Autodesk Inventor part; units mm, degrees
ref_plane "YZ Plane" through (0, 0, 0) normal (1, 0, 0) x (0, 1, 0)
ref_plane "XZ Plane" through (0, 0, 0) normal (0, 1, 0) x (-1, 0, 0)
ref_plane "XY Plane" through (0, 0, 0) normal (0, 0, 1) x (1, 0, 0)
sketch "Sketch1" plane through (0, 0, 0) normal (0, 1, 0) x (-1, 0, 0)
  line L0 (0, 0) -> (0, 27.94)
  line L1 (71.12, 27.94) -> (71.12, 0)
  arc A0 (49.5914, 27.94) -> (21.5286, 27.94) centre (35.56, 13.97) ccw
  line L2 (0, 27.94) -> (21.5286, 27.94)
  line L3 (49.5914, 27.94) -> (71.12, 27.94)
  circle A1 centre (35.56, 13.97) radius 16.5 construction
  circle A2 centre (35.56, 30.47) radius 1.5
  line L4 (35.56, 13.97) -> (49.8494, 5.72) construction
  line L5 (35.56, 13.97) -> (21.2706, 5.72) construction
  circle A3 centre (21.2706, 5.72) radius 1.5
  circle A4 centre (49.8494, 5.72) radius 1.5
  line L6 (71.12, 13.97) -> (0, 13.97) construction
  line L7 (51.7567, 0) -> (44.8805, 3.97)
  line L8 (19.3633, 0) -> (26.2395, 3.97)
  line L9 (44.8805, 3.97) -> (26.2395, 3.97)
  line L10 (59.055, 13.97) -> (64.775, 13.97) construction
  line L11 (59.055, 11.305) -> (64.775, 11.305)
  line L12 (64.775, 16.635) -> (59.055, 16.635)
  arc A5 (59.055, 16.635) -> (59.055, 11.305) centre (59.055, 13.97) ccw
  arc A6 (64.775, 11.305) -> (64.775, 16.635) centre (64.775, 13.97) ccw
  line L13 (6.33, 13.97) -> (12.08, 13.97) construction
  line L14 (6.33, 11.305) -> (12.08, 11.305)
  line L15 (12.08, 16.635) -> (6.33, 16.635)
  arc A7 (6.33, 16.635) -> (6.33, 11.305) centre (6.33, 13.97) ccw
  arc A8 (12.08, 11.305) -> (12.08, 16.635) centre (12.08, 13.97) ccw
  line L16 (71.12, 0) -> (51.7567, 0)
  line L17 (19.3633, 0) -> (0, 0)
  point P0 (61.915, 13.97)
  point P1 (9.205, 13.97)
  dimension "d0" = 27.94
  dimension "d1" = 71.12
  dimension "d5" = 35.56
  dimension "d7" = 19.8
  dimension "d8" = 33
  dimension "d9" = 3
  dimension "d10" = 3
  dimension "d11" = 3
  dimension "d13" = 30
  dimension "d14" = 4
  dimension "d15" = 4
  dimension "d16" = 10
  dimension "d17" = 2.86
  dimension "d18" = 5.33
  dimension "d19" = 2.875
  dimension "d20" = 5.33
  dimension "d21" = 26.355
  dimension "d22" = 26.355
  dimension "d23" = 13.97
extrude "Extrusion1" add sketch "Sketch1" along normal blind 4.763
fillet "Fillet1" radius 6.35 10 edges at (0, 2.3815, 0) (0, 2.3815, 27.94) (-71.12, 2.3815, 0) (-71.12, 2.3815, 27.94) (-21.5286, 2.3815, 27.94) (-49.5914, 2.3815, 27.94) (-26.2395, 2.3815, 3.97) (-19.3633, 2.3815, 0) (-44.8805, 2.3815, 3.97) (-51.7567, 2.3815, 0)
sketch "Sketch2" plane through (0, 4.763, 0) normal (0, 1, 0) x (1, 0, 0)
  arc A0 (-48.0228, -29.3557) -> (-23.0972, -29.3557) centre (-35.56, -13.97) ccw
  circle A1 centre (-35.56, -13.97) radius 3.4
  point P0 (0, 0)
  dimension "d27" = 6.8
extrude "Extrusion2" cut sketch "Sketch2" against normal blind 3
sketch "Sketch3" plane through (-35.56, 1.763, 13.97) normal (0, 1, 0) x (1, 0, 0)
  circle A0 centre (0, 0) radius 3.4
  circle A1 centre (0, 0) radius 1.75
  point P0 (35.56, 13.97)
  dimension "d30" = 3.5
extrude "Extrusion3" cut sketch "Sketch3" against normal blind 6.75 contours A1
properties part number "MountPlate"
The listing builds one solid part. Answer for the finished solid, in the listing's coordinates (mm). A direction names the side the tool comes from. Round coordinates to 2 decimals unless told otherwise and drop trailing zeros. Order: outer loops, then holes, each group sorted by start corner. A loop starts at its lowest first (then second) coordinate and runs counter-clockwise, first axis right, second up. Notation, with made-up numbers: M -28,19.25 L 31,19.25 A27 cw 31,40.25 Z; hole C 59.25,-28.75 d3. An arc over 180 degrees is marked long. Answer in a Markdown table with one row per item. Add a question column.
1) Flat-ended cylindrical pins translate along their axes: pin 1 Ø4.5 at (x, z) = (-35.56, 13.97) entering from +Y; pin 2 Ø2.5 at (x, y) = (-62, 2.5) entering from +Z; pin 3 Ø2 at (x, y) = (-30.5, 2) entering from +Z. Find the tip coordinate at first contact, or state that the pin passes through.
2) The part is cut by section A-A on x = -64. Determine the outline of the cut face in (y, z) (3 decimals).
3) Consider line 1 along X through (y, z) = (3.1, 13.97) (3 decimals); line 2 along Z through (x, y) = (-9, 4.2) (3 decimals); line 3 along X through (y, z) = (4.15, 13.5). Determine where each line is inside the solid, lowest interval first. Write a range as from..to.
4) The part is cut by section B-B on z = 13.97. Determine the outline of the cut face in (x, y) (3 decimals), plus the area to 3 significant figures.
5) Determine the mould class of faces 1 (the face through (-62, 2, 16.635)), 2 (the face through (-13, 2, 27.94)), 3 (the face through (-22.774, 2.348, 1.969)) for opening direction Z: pulls with the +Z half, pulls with the -Z half, needs draft (parallel to the pull), parting line crosses it, or undercut.
6) The part is cut by section D-D on z = 30.47. Determine the outline of the cut face in (x, y).
7) The part is cut by section C-C on y = 3.85. Count the separate pieces of the cut face and the enclosed holes in it, plus the area to 3 significant figures.
8) Which of the six approach directions +Z, -Z, +X, -X, +Y, -Y give full straight-line access (tool end or side, diameter ignored) to faces 4 (the face through (-32.42, 3.28, 15.27)), 5 (the face through (-9, 2, 16.635)), 6 (the face through (-51.792, 2.415, 0.222))?
Findings below:
| question | item | result |
|---|---|---|
| 1 | pin 1 | stops at y = 1.76 |
| 1 | pin 2 | stops at z = 27.94 |
| 1 | pin 3 | stops at z = 33.35 |
| 2 | outline | M 0,0 L 4.763,0 L 4.763,11.305 L 0,11.305 Z; M 0,16.635 L 4.763,16.635 L 4.763,27.94 L 0,27.94 Z |
| 3 | line 1 | x = -71.12..-67.44, -56.39..-38.96, -32.16..-14.745, -3.665..0 |
| 3 | line 2 | z = 0..11.305, 16.635..27.94 |
| 3 | line 3 | x = -71.12..-67.4, -56.43..-38.93, -32.19..-14.7, -3.71..0 |
| 4 | outline | M -71.12,0 L -67.44,0 L -67.44,4.763 L -71.12,4.763 Z; M -56.39,0 L -37.31,0 L -37.31,1.763 L -38.96,1.763 L -38.96,4.763 L -56.39,4.763 Z; M -33.81,0 L -14.745,0 L -14.745,4.763 L -32.16,4.763 L -32.16,1.763 L -33.81,1.763 Z; M -3.665,0 L 0,0 L 0,4.763 L -3.665,4.763 Z |
| 4 | area | 207 mm² |
| 5 | face 1 | undercut |
| 5 | face 2 | pulls with the +Z half |
| 5 | face 3 | pulls with the -Z half |
| 6 | outline | M -46.5,0 L -37.06,0 L -37.06,4.76 L -46.5,4.76 Z; M -34.06,0 L -24.62,0 L -24.62,4.76 L -34.06,4.76 Z |
| 7 | separate pieces | 1 |
| 7 | enclosed holes | 6 |
| 7 | area | 1,800 mm² |
| 8 | face 4 | +Y |
| 8 | face 5 | +Y, -Y |
| 8 | face 6 | -Z, +Y, -Y |
